Geometry: final body of the model. Coordinates: model frame, mm. A direction names the side the tool comes from. Coordinates: 2 decimals unless noted, no trailing zeros. Order: outer loops, then holes, each group sorted by start corner. A loop starts at its lowest first (then second) coordinate and runs counter-clockwise, first axis right, second up. Notation, with made-up numbers: M 35,-15.75 L 42,-15.75 A18 ccw 42,-2.75 Z; hole C 4,32.5 d4. An arc over 180 degrees is marked long. Use CSV: the item, a comma, the result in double quotes. Start each with the question number.
Q1. Section query D-D, the plane y = 1. Output: boundary loops of the cut face in (x, z), and give its area (3 significant figures).
Q2. Section query C-C, the plane x = 26. Output: boundary loops of the cut face in (y, z), and give its area (3 significant figures).
Q3. First-contact query: P1, Ø0.5, axis at x = -21.5, z = 2.5, coming from the +Y side; P2, Ø10, axis at x = 9, y = 7.5, coming from the -Z side; P3, Ø1.5, axis at x = 26.5, z = 2, coming from the -Y side. Flat tips, straight axial feed; report the tip coordinate or a pass-through.
Q4. Section query A-A, the plane z = 0.7. Output: boundary loops of the cut face in (x, y), and give its area (3 significant figures).
Q5. Ray query, probe 1 along Y at (x, z) = (-9.5, 2.5); probe 2 along X at (y, z) = (-4, 2.35); probe 3 along X at (y, z) = (10, 2.7). Return the intervals inside material, ascending.
Q6. Section query B-B, the plane x = 15.5. Output: boundary loops of the cut face in (y, z), and give its area (3 significant figures).
Q7. Access query for faces 1 (the face through (30, 11.711, 1)), 2 (the face through (2.645, 7.861, 2.493)), 3 (the face through (1, -2, 0)). Directions: +Z, -Z, +X, -X, +Y, -Y. A direction counts if a zero-diameter tool reaches every point of the face in a straight line with its end or side. Return the directions, or none.
Q8. Mould query, pull axis Y, two halves, no side actions, for faces 4 (the face through (-8, -17.389, 1)), 5 (the face through (26.638, 5.855, 1.479)), 6 (the face through (13, -1, 3)), 7 (the face through (33.31, 6.02, 1.48)). Classes: +Y half, -Y half, draft (parallel to the pull), parting line (faces both ways), or undercut.
from build123d import *

# Parameters (mm, degrees)
F1_DEPTH = 2
F2_DEPTH = 3


with BuildPart() as f1:
    # F0 (on Top) → F1 (new body)
    with BuildSketch(Plane.XY):
        Polygon((-18.2464108846, 11.7113475275), (-33.8927962614, -15.3889868999), (-13.4678907388, -15.3889868999), (-15.2466582433, -5.3010950903), (-23.0469053902, -5.3010950903), (-23.6242556594, -4.3010950903), (-23.0469053902, -3.3010950903), (-15.5993122047, -3.3010950903), align=None)
    extrude(amount=F1_DEPTH)



with BuildPart() as f1b:
    # F0 (on Top) → F1, piece 2 (new body)
    with BuildSketch(Plane.XY):
        Polygon((-16.2464108846, 11.7113475275), (-11.4678907388, -15.3889868999), (-0.5617896535, -15.3889868999), (1.4382103465, -15.3889868999), (1.7851558166, -15.3889868999), (-0.5617896535, -2.078797724), (-8.5276595022, -2.078797724), (-9.1050097714, -1.078797724), (-8.5276595022, -0.078797724), (1.4382103465, -0.078797724), (4.137809778, -15.3889868999), (20.9472483989, -15.3889868999), (28.7704410873, -1.8388196862), (20.9472483989, 11.7113475275), (4.8681087356, 11.7113475275), (0.4830753681, 4.1162469421), (-0.6402473631, 3.8304019006), (-8.3246870782, 11.7113475275), align=None)
        Polygon((19.4851677419, -0.8388196862), (18.9078174727, -1.8388196862), (8.0837683482, -1.8388196862), (7.5064180791, -0.8388196862), (8.0837683482, 0.1611803138), (18.9078174727, 0.1611803138), align=None, mode=Mode.SUBTRACT)
    extrude(amount=F1_DEPTH)


with BuildPart() as f1_1:
    add(f1.part)

    add(f1b.part)  # F2 merges F1b
    # F0 (on Top) → F2 (join)
    with BuildSketch(Plane.XY):
        Polygon((22.1019489373, 13.7113475275), (-19.401111423, 13.7113475275), (-37.3568978765, -17.3889868999), (-13.9558746851, -17.3889868999), (22.1019489373, -17.3889868999), (31.079842164, -1.8388196862), (40.0577353908, 13.7113475275), align=None)
        Polygon((-13.4678907388, -15.3889868999), (-33.8927962614, -15.3889868999), (-18.2464108846, 11.7113475275), (-16.2464108846, 11.7113475275), (-8.3246870782, 11.7113475275), (-5.5734554462, 11.7113475275), (4.8681087356, 11.7113475275), (20.9472483989, 11.7113475275), (28.7704410873, -1.8388196862), (20.9472483989, -15.3889868999), (4.137809778, -15.3889868999), (1.7851558166, -15.3889868999), (1.4382103465, -15.3889868999), (-0.5617896535, -15.3889868999), (-11.4678907388, -15.3889868999), align=None, mode=Mode.SUBTRACT)
        Polygon((36.5936337757, 11.7113475275), (29.9251416257, 0.1611803138), (23.2566494757, 11.7113475275), align=None, mode=Mode.SUBTRACT)
        Polygon((-23.0469053902, -5.3010950903), (-15.2466582433, -5.3010950903), (-15.5993122047, -3.3010950903), (-23.0469053902, -3.3010950903), (-23.6242556594, -4.3010950903), align=None)
        Polygon((-15.2466582433, -5.3010950903), (-13.4678907388, -15.3889868999), (-11.4678907388, -15.3889868999), (-16.2464108846, 11.7113475275), (-18.2464108846, 11.7113475275), (-15.5993122047, -3.3010950903), align=None)
        Polygon((-0.5617896535, -2.078797724), (1.7851558166, -15.3889868999), (4.137809778, -15.3889868999), (1.4382103465, -0.078797724), (-8.5276595022, -0.078797724), (-9.1050097714, -1.078797724), (-8.5276595022, -2.078797724), align=None)
        Polygon((-5.5734554462, 11.7113475275), (-8.3246870782, 11.7113475275), (-0.6402473631, 3.8304019006), (0.4830753681, 4.1162469421), (0.7917058952, 5.2266503978), align=None)
        Polygon((4.8681087356, 11.7113475275), (-5.5734554462, 11.7113475275), (0.7917058952, 5.2266503978), (0.4830753681, 4.1162469421), align=None)
        Polygon((8.0837683482, -1.8388196862), (18.9078174727, -1.8388196862), (19.4851677419, -0.8388196862), (18.9078174727, 0.1611803138), (8.0837683482, 0.1611803138), (7.5064180791, -0.8388196862), align=None)
    extrude(amount=F2_DEPTH)


solid = f1_1.part
Responses:
1,outline,"M -26.74,0 L 29.44,0 L 29.44,3 L 27.13,3 L 27.13,2 L -14.36,2 L -14.36,3 L -16.36,3 L -16.36,2 L -24.43,2 L -24.43,3 L -26.74,3 Z; M 30.41,0 L 32.72,0 L 32.72,3 L 30.41,3 Z"
1,area,"126 mm²"
2,outline,"M -10.64,0 L 6.96,0 L 6.96,3 L 2.96,3 L 2.96,2 L -6.64,2 L -6.64,3 L -10.64,3 Z; M 11.71,0 L 13.71,0 L 13.71,3 L 11.71,3 Z"
2,area,"49.2 mm²"
3,P1,"stops at y = 10.51"
3,P2,"stops at z = 0"
3,P3,"stops at y = -11.07"
4,outline,"M -37.36,-17.39 L 22.1,-17.39 L 40.06,13.71 L -19.4,13.71 Z; hole M 23.26,11.71 L 29.93,0.16 L 36.59,11.71 Z"
4,area,"1,770 mm²"
5,probe 1,"y = -17.39 to -15.39, 11.71 to 13.71"
5,probe 2,"x = -29.63 to -27.32, -23.45 to -13.48, -0.22 to 2.13, 27.52 to 29.83"
5,probe 3,"x = -21.54 to -19.23, -17.94 to -15.94, -6.66 to 3.88, 21.94 to 24.24, 35.61 to 37.91"
6,outline,"M -17.39,0 L 13.71,0 L 13.71,3 L 11.71,3 L 11.71,2 L 0.16,2 L 0.16,3 L -1.84,3 L -1.84,2 L -15.39,2 L -15.39,3 L -17.39,3 Z"
6,area,"68.2 mm²"
7,face 1,"+Z, -Z"
7,face 2,"+Z"
7,face 3,"-Z, +X, -X, +Y, -Y"
8,face 4,"-Y half"
8,face 5,"undercut"
8,face 6,"draft"
8,face 7,"undercut"
